Answer from the drawing. Dimensions are ordinates in mm from the lowest x, y and z of the part. A direction names the side the tool comes from. Coordinates: 2 decimals unless noted, no trailing zeros. Write each loop counter-clockwise with the first axis right and the second up, starting at its lowest first coordinate (ties: lowest second). Pieces come first, ordered by that corner, then holes. Notation, with made-up numbers: (86, 4.5) - (115, 4.5) arc R17 cw to (115, 9.5) - close; hole circle Ø8 at (17.25, 13). An arc over 180 degrees is marked (long way). Return JSON: item names as keys, results as strings.
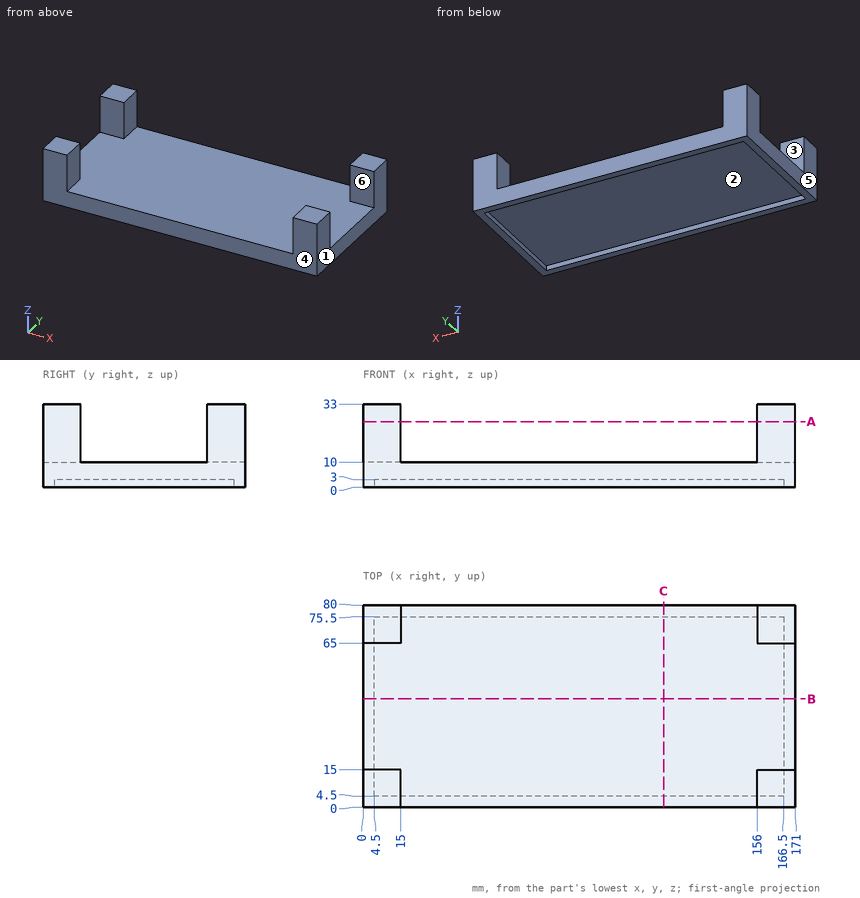
(1) A cutting plane is placed at B-B (y = 43). Determine the outline of the cut face in (x, z), and give its area (3 significant figures).
Answer:
{"outline": "(0, 0) - (4.5, 0) - (4.5, 3) - (166.5, 3) - (166.5, 0) - (171, 0) - (171, 10) - (0, 10) - close", "area": "1,220 mm²"}
(2) Straight lines are drawn through the part: line 1 (Y direction, x = 17, z = 2); line 2 (Z direction, x = 134.5, y = 57); line 3 (X direction, y = 66, z = 31.5). For each, find the intervals that lie inside material, in ascending order. Write a range as from..to.
Answer:
{"line 1": "0..4.5, 75.5..80", "line 2": "3..10", "line 3": "0..15, 156..171"}
(3) A cutting plane is placed at A-A (z = 26). Determine the outline of the cut face in (x, y).
Answer:
{"outline": "(0, 0) - (15, 0) - (15, 15) - (0, 15) - close; (0, 65) - (15, 65) - (15, 80) - (0, 80) - close; (156, 0) - (171, 0) - (171, 15) - (156, 15) - close; (156, 65) - (171, 65) - (171, 80) - (156, 80) - close"}
(4) Determine the mould class of the marked faces 4, 5 and 6 for opening direction Y: +Y half, -Y half, draft (parallel to the pull), parting line (faces both ways), or undercut.
Answer:
{"face 4": "-Y half", "face 5": "draft", "face 6": "undercut"}
(5) Which of the six approach directions +Z, -Z, +X, -X, +Y, -Y give full straight-line access (tool end or side, diameter ignored) to the marked faces 1, 2 and 3?
Answer:
{"face 1": "+Z, -Z, +X, +Y, -Y", "face 2": "-Z", "face 3": "+Z, +X, -X"}
(6) Flat-ended cylindrical pins translate along their axes: P1, Ø24, axis at x = 112.5, y = 36, coming from the +Z side; P2, Ø1, axis at x = 152.5, y = 54.5, coming from the -Z side. Find the tip coordinate at first contact, or state that the pin passes through.
Answer:
{"P1": "z = 10", "P2": "z = 3"}
(7) A cutting plane is placed at C-C (x = 119). Determine the outline of the cut face in (y, z), and give its area (3 significant figures).
Answer:
{"outline": "(0, 0) - (4.5, 0) - (4.5, 3) - (75.5, 3) - (75.5, 0) - (80, 0) - (80, 10) - (0, 10) - close", "area": "587 mm²"}
